Source: three-view drawing plus pictorial views. Frame: mm from the lowest corner of the part. A direction names the side the tool comes from. Give positions to 0.01 mm unless a question says otherwise; leave off trailing zeros. Loops run counter-clockwise (first coordinate to the right, second up) from the corner with the lowest first, then second, coordinate; pieces in that order, holes last. Notation, with made-up numbers: (-4.75, 57) - (-0.75, 57) arc R31 ccw to (-0.75, 87) - close; hole circle Ø7 at (29.5, 72). An arc over 180 degrees is marked (long way). Answer in a Markdown table with one row per item.
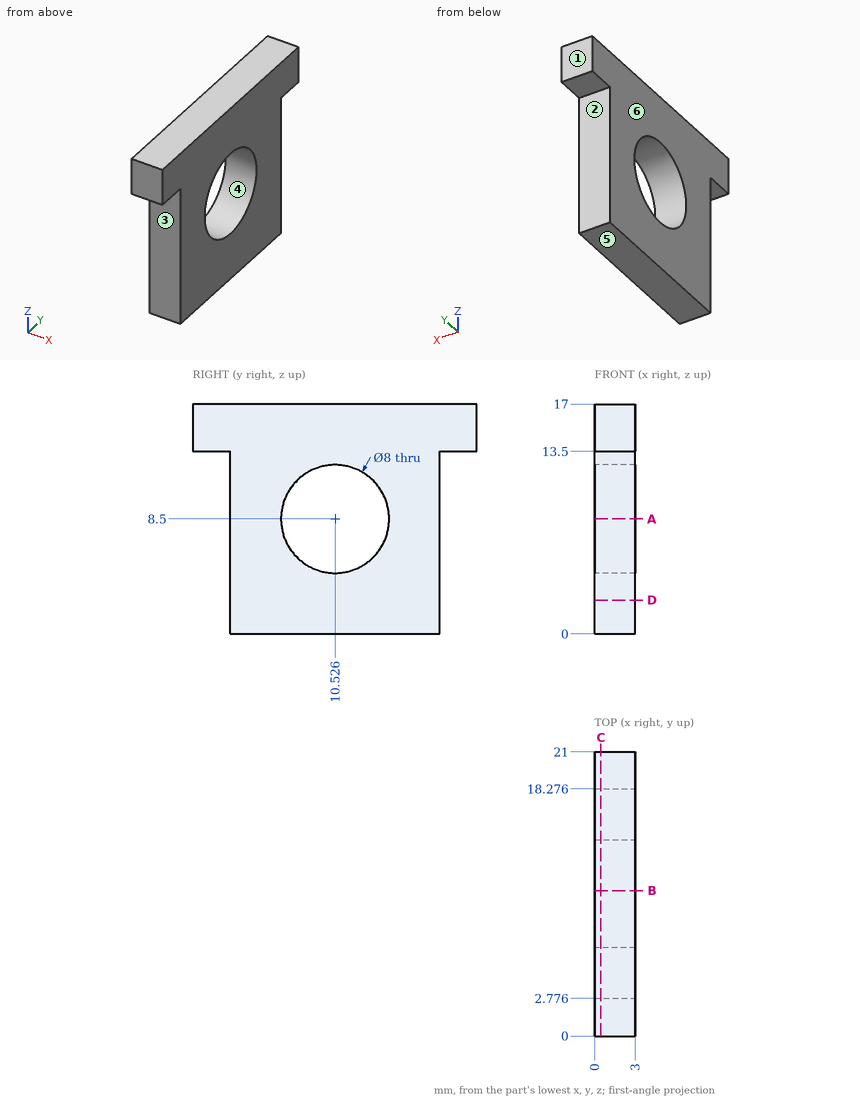
Q1. First-contact query: pin 1 (0.9 mm diameter, centred on x = 1, z = 8, fed in from -Y); pin 2 (0.8 mm diameter, centred on x = 1, y = 2, fed in from -Z). Flat tips, straight axial feed; report the tip coordinate or a pass-through.
Check values:
| item | result |
|---|---|
| pin 1 | y = 2.78 |
| pin 2 | z = 13.5 |
Q2. Cut plane C-C (x = 0.45). Output: boundary loops of the cut face in (y, z).
Check values:
| item | result |
|---|---|
| outline | (0, 13.5) - (2.78, 13.5) - (2.78, 0) - (18.28, 0) - (18.28, 13.5) - (21, 13.5) - (21, 17) - (0, 17) - close; hole circle Ø8 at (10.53, 8.5) |
Q3. Cut plane A-A (z = 8.5). Output: boundary loops of the cut face in (x, y).
Check values:
| item | result |
|---|---|
| outline | (0, 2.78) - (3, 2.78) - (3, 6.53) - (0, 6.53) - close; (0, 14.53) - (3, 14.53) - (3, 18.28) - (0, 18.28) - close |
Q4. Draft query along Z for the marked faces 4, 5 and 6. Return one class per face: pulls with the +Z half, pulls with the -Z half, needs draft (parallel to the pull), parting line crosses it, or undercut.
Check values:
| item | result |
|---|---|
| face 4 | undercut |
| face 5 | pulls with the -Z half |
| face 6 | needs draft |
Q5. Cut plane B-B (y = 10.75). Output: boundary loops of the cut face in (x, z).
Check values:
| item | result |
|---|---|
| outline | (0, 0) - (3, 0) - (3, 4.51) - (0, 4.51) - close; (0, 12.49) - (3, 12.49) - (3, 17) - (0, 17) - close |
Q6. Cut plane D-D (z = 2.5). Output: boundary loops of the cut face in (x, y).
Check values:
| item | result |
|---|---|
| outline | (0, 2.78) - (3, 2.78) - (3, 18.28) - (0, 18.28) - close |
Q7. Reachability of the marked faces 1, 2 and 3 from +Z, -Z, +X, -X, +Y, -Y: full face, straight path, thin tool, end or side. Return the list, or none.
Check values:
| item | result |
|---|---|
| face 1 | +Z, -Z, +X, -X, +Y |
| face 2 | -Z, +X, -X, +Y |
| face 3 | -Z, +X, -X, -Y |
Q8. Material intervals for line 1 along Y through (x, z) = (1.05, 2); line 2 along Z through (x, y) = (2.1, 14); line 3 along Y through (x, z) = (0.55, 6), sorted ascending.
Check values:
| item | result |
|---|---|
| line 1 | 2.78 to 18.28 |
| line 2 | 0 to 6.52, 10.48 to 17 |
| line 3 | 2.78 to 7.4, 13.65 to 18.28 |
